```python
from build123d import *

# Parameters (mm, degrees)
BOSS_EXTRUDE1_DEPTH            = 7.5
BOSS_EXTRUDE1_DEPTH_BACK       = 7.5
CUT_EXTRUDE3_REACH             = 31.568
SKETCH5_R                      = 1.5
FILLET1_R                      = 5
CUT_EXTRUDE2_REACH             = 19.405
SKETCH3_R                      = 0.5
CUT_EXTRUDE2_DIRECTION_2_REACH = 19.405
FILLET2_R                      = 5
BOSS_EXTRUDE2_DEPTH            = 3.7
BOSS_EXTRUDE2_DEPTH_BACK       = 3.7
SKETCH6_R                      = 1.2


with BuildPart() as part:
    # Sketch1 → Boss-Extrude1 (new, two sides: drawn at the far end of the back side and taken through both)
    with BuildSketch(Plane(origin=(0, 0, 0), x_dir=(-1, 0, 0), z_dir=(0, 1, 0)).offset(-BOSS_EXTRUDE1_DEPTH_BACK)):
        with BuildLine():
            Line((6.3, 7.5), (-6.3, 7.5))
            Line((-6.3, 7.5), (-12.102943725, 1.697056275))
            ThreePointArc((-12.102943725, 1.697056275), (-11.582689122, -0.918440238), (-13.8, -2.4))
            Line((-13.8, -2.4), (-13.8, -7.5))
            Line((-13.8, -7.5), (13.8, -7.5))
            Line((13.8, -7.5), (13.8, -2.4))
            ThreePointArc((13.8, -2.4), (11.582689122, -0.918440238), (12.102943725, 1.697056275))
            Line((12.102943725, 1.697056275), (6.3, 7.5))
        make_face()
    extrude(amount=BOSS_EXTRUDE1_DEPTH + BOSS_EXTRUDE1_DEPTH_BACK)

    # Sketch5 → Cut-Extrude3 (cut, up to next)
    with BuildSketch(Plane.YZ.offset(13.8), mode=Mode.PRIVATE) as cut_extrude3_sk1:
        with Locations(Location((-2.25, -4.95, 0), (0, 0, 270))):
            Circle(SKETCH5_R)
    cut_extrude3_tool1 = extrude(cut_extrude3_sk1.sketch, amount=-CUT_EXTRUDE3_REACH, mode=Mode.PRIVATE) & part.part
    # Sketch5 → Cut-Extrude3 (cut, up to next)
    with BuildSketch(Plane.YZ.offset(13.8), mode=Mode.PRIVATE) as cut_extrude3_sk2:
        with Locations(Location((2.25, -4.95, 0), (0, 0, 270))):
            Circle(SKETCH5_R)
    cut_extrude3_tool2 = extrude(cut_extrude3_sk2.sketch, amount=-CUT_EXTRUDE3_REACH, mode=Mode.PRIVATE) & part.part
    add(cut_extrude3_tool1.solids().sort_by_distance((13.8, -2.25, -4.95))[0], mode=Mode.SUBTRACT)
    add(cut_extrude3_tool2.solids().sort_by_distance((13.8, 2.25, -4.95))[0], mode=Mode.SUBTRACT)

    # Fillet1
    fillet1_edges = [part.edges().sort_by_distance(p)[0] for p in [
        (0, -7.5, -7.5),
        (0, 7.5, -7.5),
    ]]
    fillet(fillet1_edges, radius=FILLET1_R)

    # Cut-Extrude2: up to this plane
    cut_extrude2_end = Plane(origin=(-6.9, -7.5, 6.9), z_dir=(0.7071067811865475, 0, -0.7071067811865477))
    # Sketch3 → Cut-Extrude2 (cut, up to the surface)
    with BuildSketch(Plane.YZ, mode=Mode.PRIVATE) as cut_extrude2_sk1:
        with Locations(Location((0, 4.598528137, 0), (0, 0, 90))):
            Circle(SKETCH3_R)
    cut_extrude2_tool1 = split(extrude(cut_extrude2_sk1.sketch, amount=-CUT_EXTRUDE2_REACH, mode=Mode.PRIVATE), bisect_by=cut_extrude2_end, keep=Keep.BOTH, mode=Mode.PRIVATE)
    add(cut_extrude2_tool1.solids().sort_by_distance((0, 0, 4.598528))[0], mode=Mode.SUBTRACT)

    # Cut-Extrude2 direction 2: up to this plane
    cut_extrude2_direction_2_end = Plane(origin=(6.9, -7.5, 6.9), z_dir=(-0.7071067811865475, 0, -0.7071067811865476))
    # Sketch3 → Cut-Extrude2 direction 2 (cut, up to the surface)
    with BuildSketch(Plane.YZ, mode=Mode.PRIVATE) as cut_extrude2_direction_2_sk1:
        with Locations(Location((0, 4.598528137, 0), (0, 0, 90))):
            Circle(SKETCH3_R)
    cut_extrude2_direction_2_tool1 = split(extrude(cut_extrude2_direction_2_sk1.sketch, amount=CUT_EXTRUDE2_DIRECTION_2_REACH, mode=Mode.PRIVATE), bisect_by=cut_extrude2_direction_2_end, keep=Keep.BOTH, mode=Mode.PRIVATE)
    add(cut_extrude2_direction_2_tool1.solids().sort_by_distance((0, 0, 4.598528))[0], mode=Mode.SUBTRACT)

    # Fillet2
    fillet2_edges = [part.edges().sort_by_distance(p)[0] for p in [
        (0, 7.5, 7.5),
        (0, -7.5, 7.5),
    ]]
    fillet(fillet2_edges, radius=FILLET2_R)

    # Sketch6 → Boss-Extrude2 (add, two sides: drawn at the far end of the back side and taken through both)
    # profile 1 of 2: a face of its own
    with BuildSketch(Plane(origin=(0, 0, 0), x_dir=(-1, 0, 0), z_dir=(0, 1, 0)).offset(-BOSS_EXTRUDE2_DEPTH_BACK)):
        with BuildLine():
            Line((-12.102943725, 1.697056275), (-12.244365081, 1.555634919))
            ThreePointArc((-12.244365081, 1.555634919), (-15.832534972, 0.841903551), (-13.8, -2.2))
            Line((-13.8, -2.2), (-13.8, -2.4))
            ThreePointArc((-13.8, -2.4), (-11.582689122, -0.918440238), (-12.102943725, 1.697056275))
        make_face()
        with Locations(Location((-13.8, 0, 0), (0, 0, 90))):
            Circle(SKETCH6_R, mode=Mode.SUBTRACT)
    # profile 2 of 2: a face of its own
    with BuildSketch(Plane(origin=(0, 0, 0), x_dir=(-1, 0, 0), z_dir=(0, 1, 0)).offset(-BOSS_EXTRUDE2_DEPTH_BACK)):
        with BuildLine():
            Line((13.8, -2.4), (13.8, -2.2))
            ThreePointArc((13.8, -2.2), (15.832534972, 0.841903551), (12.244365081, 1.555634919))
            Line((12.244365081, 1.555634919), (12.102943725, 1.697056275))
            ThreePointArc((12.102943725, 1.697056275), (11.582689122, -0.918440238), (13.8, -2.4))
        make_face()
        with Locations(Location((13.8, 0, 0), (0, 0, 270))):
            Circle(SKETCH6_R, mode=Mode.SUBTRACT)
    extrude(amount=BOSS_EXTRUDE2_DEPTH + BOSS_EXTRUDE2_DEPTH_BACK)


solid = part.part
```
CAD build for the part. Positions are in the model's coordinates, mm. A direction names the side the tool comes from. Round coordinates to 2 decimals unless told otherwise and drop trailing zeros. Loops run counter-clockwise (first coordinate to the right, second up) from the corner with the lowest first, then second, coordinate; pieces in that order, holes last. Notation, with made-up numbers: M 10,-30.75 L 66,-30.75 A35 cw 66,7.25 Z; hole C 66.5,-8.75 d3. An arc over 180 degrees is marked long. Return JSON: item names as keys, results as strings. Group by question number.
(1) Drop flat-ended pins along their axis: P1, Ø1.9, axis at x = -13.8, z = 0, coming from the -Y side; P2, Ø6, axis at x = 9.5, y = 3.5, coming from the +Z side; P3, Ø2, axis at y = -4, z = -4, coming from the +X side; P4, Ø1, axis at y = 6, z = 6, coming from the +X side. Give the stop position or say it passes through.
(2) Wall check: probe 1 along X at (y, z) = (1, 0); probe 2 along Y at (x, z) = (1.75, -4.95); probe 3 along X at (y, z) = (-2, -3). Give the ranges that are in metal, low to high. Write a range as [from, to].
(3) Saw through at C-C, the plane x = 13. List the corners of the cut face in (y, z), and give its area (3 significant figures).
(4) Saw through at D-D, the plane x = 1.5. List the corners of the cut face in (y, z).
(5) Mould opens along Z. For faces 1 (the cylindrical face through (-0.19, 6.07, -6)), 2 (the cylindrical face through (-15.855, -0.052, 0.786)), 3 (the cylindrical face through (11.568, 5.573, -0.882)) say: +Z half, -Z half, draft (parallel to the pull), parting line (faces both ways), or undercut.
(6) Saw through at B-B, the plane y = 0. List the corners of the cut face in (x, z).
(7) Tool access for faces 4 (the flat face through (13.8, 0, -4)), 5 (the cylindrical face through (-11.598, 5.573, -0.955)), 6 (the flat face through (0, 7.5, 0)), 7 (the cylindrical face through (-11.598, -5.627, -0.955)), 8 (the flat face through (0, 0, 7.5)): list every direction of +Z, -Z, +X, -X, +Y, -Y with a clear straight run to the whole face (end or side of a thin tool).
(8) Saw through at A-A, the plane z = 0. List the corners of the cut face in (x, y).
Answer list:
{
 "1": {"P1": "through", "P2": "z = 7.3", "P3": "x = 13.8", "P4": "x = 8.3"},
 "2": {"probe 1": "[-16, -15], [-12.6, 12.6], [15, 16]", "probe 2": "[-6.86, -3.75], [-0.75, 0.75], [3.75, 6.86]", "probe 3": "[-13.8, 13.8]"},
 "3": {"outline": "M -7.5,-2.5 A5 ccw -2.5,-7.5 L 2.5,-7.5 A5 ccw 7.5,-2.5 L 7.5,-2.26 L 3.7,-2.26 L 3.7,-0.89 L -3.7,-0.89 L -3.7,-2.26 L -7.5,-2.26 Z; M -3.7,0.89 L 3.7,0.89 L 3.7,2.05 L -3.7,2.05 Z; hole C -2.25,-4.95 d3; hole C 2.25,-4.95 d3", "area": "72.4 mm2"},
 "4": {"outline": "M -7.5,-2.5 A5 ccw -2.5,-7.5 L 2.5,-7.5 A5 ccw 7.5,-2.5 L 7.5,2.5 A5 ccw 2.5,7.5 L -2.5,7.5 A5 ccw -7.5,2.5 Z; hole C -2.25,-4.95 d3; hole C 0,4.6 d1; hole C 2.25,-4.95 d3"},
 "5": {"face 1": "-Z half", "face 2": "parting line", "face 3": "undercut"},
 "6": {"outline": "M -13.8,-7.5 L 13.8,-7.5 L 13.8,-2.2 A2.2 ccw long 12.24,1.56 L 9.7,4.1 L -9.7,4.1 L -12.24,1.56 A2.2 ccw long -13.8,-2.2 Z; M -8.7,5.1 L 8.7,5.1 L 6.3,7.5 L -6.3,7.5 Z; hole C -13.8,0 d2.4; hole C 13.8,0 d2.4"},
 "7": {"face 4": "-Z, +X, +Y, -Y", "face 5": "-X, +Y", "face 6": "+Z, -Z, +X, -X, +Y", "face 7": "-X, -Y", "face 8": "+Z, +X, -X, +Y, -Y"},
 "8": {"outline": "M -16,-3.7 L -15,-3.7 L -15,3.7 L -16,3.7 Z; M -12.6,-3.7 L -11.4,-3.7 L -11.4,-7.5 L 11.4,-7.5 L 11.4,-3.7 L 12.6,-3.7 L 12.6,3.7 L 11.4,3.7 L 11.4,7.5 L -11.4,7.5 L -11.4,3.7 L -12.6,3.7 Z; M 15,-3.7 L 16,-3.7 L 16,3.7 L 15,3.7 Z"}
}
